For this review, take the finished solid that the model builds, in its own axes (mm). A direction names the side the tool comes from. Round coordinates to 2 decimals unless told otherwise and drop trailing zeros. Order: outer loops, then holes, each group sorted by start corner. A loop starts at its lowest first (then second) coordinate and runs counter-clockwise, first axis right, second up. Notation, with made-up numbers: M -35,-18 L 19,-18 A33 cw 19,13 Z; hole C 24,74 d8. An arc over 180 degrees is marked long. Use a Markdown table: item, result.
from build123d import *

# Parameters (mm, degrees)
F0_W     = 47
F0_H     = 2
F0_W_2   = 10
F0_H_2   = 3.4
F1_DEPTH = 4
F2_DEPTH = 10
F3_R     = 1


with BuildPart() as f1:
    # F0 (on Top) → F1 (new body)
    with BuildSketch(Plane.XY):
        with Locations((-12.59553, 9.557682)):
            Rectangle(F0_W, F0_H)
        Polygon((10.90447, 10.657682), (10.90447, 10.557682), (10.90447, 8.557682), (10.90447, 3.057682), (32.90447, 3.057682), (32.90447, 14.057682), (20.90447, 14.057682), (20.90447, 10.657682), align=None)
        with Locations((15.90447, 12.357682)):
            Rectangle(F0_W_2, F0_H_2)
    extrude(amount=F1_DEPTH)

    # F0 (on Top) → F2 (join)
    with BuildSketch(Plane.XY):
        with Locations((15.90447, 12.357682)):
            Rectangle(F0_W_2, F0_H_2)
    extrude(amount=F2_DEPTH)

    # F3
    f3_edges = [f1.edges().sort_by_distance(p)[0] for p in [
        (32.90447, 3.057682, 2),
        (32.90447, 14.057682, 2),
    ]]
    fillet(f3_edges, radius=F3_R)


solid = f1.part
Q1. Add section D-D (z = 6). Write out the cut boundary in (x, y), then the cut area to 3 significant figures.
Determined:
| item | result |
|---|---|
| outline | M 10.9,10.66 L 20.9,10.66 L 20.9,14.06 L 10.9,14.06 Z |
| area | 34.0 mm^2 |
Q2. Machinability: for faces 1 (the flat face through (10.904, 6, 2)), 2 (the flat face through (16, 10.658, 7)), 3 (the flat face through (19, 14.058, 4)), 4 (the flat face through (20.904, 12, 7)), 5 (the flat face through (10.904, 12, 5)), which of the approach directions +Z, -Z, +X, -X, +Y, -Y give a long, thin tool a straight path to every point of the face, cutting with its end or side? Answer none if there is none.
Determined:
| item | result |
|---|---|
| face 1 | +Z, -Z, -X, -Y |
| face 2 | +Z, +X, -X, -Y |
| face 3 | +Z, -Z, +X, -X, +Y |
| face 4 | +Z, +X, +Y, -Y |
| face 5 | +Z, -Z, -X, +Y |
Q3. Add section B-B (z = 3). Write out the cut boundary in (x, y), then the cut area to 3 significant figures.
Determined:
| item | result |
|---|---|
| outline | M -36.1,8.56 L 10.9,8.56 L 10.9,3.06 L 31.9,3.06 A1 ccw 32.9,4.06 L 32.9,13.06 A1 ccw 31.9,14.06 L 10.9,14.06 L 10.9,10.56 L -36.1,10.56 Z |
| area | 336 mm^2 |
Q4. Wall thickness on line 1 along Z through (x, y) = (15.5, 8.5); line 2 along Y through (x, z) = (-13.5, 1.5); line 3 along Y through (x, z) = (20, 7.5): over which ranges is each line inside the solid? List them lowest first. Write a range as [from, to].
Determined:
| item | result |
|---|---|
| line 1 | z = [0, 4] |
| line 2 | y = [8.56, 10.56] |
| line 3 | y = [10.66, 14.06] |
Q5. Clearance check with flat-ended pins moving along their axes: pin 1 (1 mm diameter, centred on y = 6.5, z = 5.5, fed in from +X); pin 2 (5 mm diameter, centred on y = 12.5, z = 6, fed in from -X); pin 3 (4 mm diameter, centred on x = 11.5, y = 4, fed in from +Z); pin 4 (1.8 mm diameter, centred on x = 16.5, z = 8.5, fed in from -Y). State where each tip first meets the part, or that it passes through.
Determined:
| item | result |
|---|---|
| pin 1 | passes through |
| pin 2 | stops at x = 10.9 |
| pin 3 | stops at z = 4 |
| pin 4 | stops at y = 10.66 |
Q6. Add section A-A (y = 11.25). Write out the cut boundary in (x, z).
Determined:
| item | result |
|---|---|
| outline | M 10.9,0 L 32.9,0 L 32.9,4 L 20.9,4 L 20.9,10 L 10.9,10 Z |
Q7. Add section C-C (x = 16.5). Write out the cut boundary in (y, z), then the cut area to 3 significant figures.
Determined:
| item | result |
|---|---|
| outline | M 3.06,0 L 14.06,0 L 14.06,10 L 10.66,10 L 10.66,4 L 3.06,4 Z |
| area | 64.4 mm^2 |
